Design review of the part built by this model. Coordinates are the model's own, in mm. A direction names the side the tool comes from. Coordinates: 2 decimals unless noted, no trailing zeros. Loops run counter-clockwise (first coordinate to the right, second up) from the corner with the lowest first, then second, coordinate; pieces in that order, holes last. Notation, with made-up numbers: (31.25, -12) -> (85.25, -12) arc R26 ccw to (85.25, 4) -> close; hole circle Ø10 at (-30, -10). An arc over 180 degrees is marked (long way). Answer as a JSON object with one key per item and string values.
```python
from build123d import *

# Parameters (mm, degrees)
F0_W     = 70.104
F0_H     = 85.09
F1_DEPTH = 10
F2_W     = 55.88
F2_H     = 85.09
F3_DEPTH = 14
F4_W     = 57.15
F4_H     = 85.09
F5_DEPTH = 10


with BuildPart() as f1:
    # F0 (on Top) → F1 (new body, symmetric)
    with BuildSketch(Plane.XY):
        Rectangle(F0_W, F0_H)
    extrude(amount=F1_DEPTH, both=True)

    # F2 (on face) → F3 (join)
    with BuildSketch(Plane.XY.offset(10)):
        Rectangle(F2_W, F2_H)
    extrude(amount=F3_DEPTH)

    # F4 (on face) → F5 (join)
    with BuildSketch(Plane.XY.offset(24)):
        Rectangle(F4_W, F4_H)
    extrude(amount=F5_DEPTH)


solid = f1.part
```
1) Add section B-B, the plane z = 29. Give the boundary of the cut face in (x, y) (3 decimals).
Completed:
{"outline": "(-28.575, -42.545) -> (28.575, -42.545) -> (28.575, 42.545) -> (-28.575, 42.545) -> close"}
2) For faces 1 (the flat face through (-28.575, -1, 29)), 2 (the flat face through (28.575, -1, 29)), 3 (the flat face through (-35.052, -1, 0)), 4 (the flat face through (-27.94, -1, 17)), 5 (the flat face through (0, 42.545, 12)), list the 3-axis set-ups (+Z, -Z, +X, -X, +Y, -Y) from which the entire face can be reached by the end or side of a thin tool; tool diameter is ignored.
Completed:
{"face 1": "+Z, -X, +Y, -Y", "face 2": "+Z, +X, +Y, -Y", "face 3": "+Z, -Z, -X, +Y, -Y", "face 4": "-X, +Y, -Y", "face 5": "+Z, -Z, +X, -X, +Y"}
3) Add section C-C, the plane z = 11.5. Give the boundary of the cut face in (x, y) (3 decimals), and give its area (3 significant figures).
Completed:
{"outline": "(-27.94, -42.545) -> (27.94, -42.545) -> (27.94, 42.545) -> (-27.94, 42.545) -> close", "area": "4,750 mm²"}
4) Add section A-A, the plane y = 30. Give the boundary of the cut face in (x, z) (3 decimals), and give its area (3 significant figures).
Completed:
{"outline": "(-35.052, -10) -> (35.052, -10) -> (35.052, 10) -> (27.94, 10) -> (27.94, 24) -> (28.575, 24) -> (28.575, 34) -> (-28.575, 34) -> (-28.575, 24) -> (-27.94, 24) -> (-27.94, 10) -> (-35.052, 10) -> close", "area": "2,760 mm²"}
5) Clearance check with flat-ended pins moving along their axes: pin 1 Ø3 at (y, z) = (3.5, 27) entering from +X (3 decimals); pin 2 Ø3.5 at (x, y) = (32.5, -8) entering from +Z; pin 3 Ø7 at (y, z) = (8, 20) entering from +X. State where each tip first meets the part, or that it passes through.
Completed:
{"pin 1": "x = 28.575", "pin 2": "z = 10", "pin 3": "x = 27.94"}
6) Wall thickness on probe 1 along Z at (x, y) = (-28.5, -2); probe 2 along Z at (x, y) = (30, 26); probe 3 along X at (y, z) = (-10, 28.5) (3 decimals): over which ranges is each line inside the solid? List them lowest first.
Completed:
{"probe 1": "-10 to 10, 24 to 34", "probe 2": "-10 to 10", "probe 3": "-28.575 to 28.575"}
7) The part is to be moulded in two halves that separate along Z. For faces 6 (the flat face through (0, 1, -10)), 7 (the flat face through (27.94, -1, 17)), 8 (the flat face through (0, -42.545, 12)), say which applies: pulls with the +Z half, pulls with the -Z half, needs draft (parallel to the pull), parting line crosses it, or undercut.
Completed:
{"face 6": "pulls with the -Z half", "face 7": "undercut", "face 8": "needs draft"}
